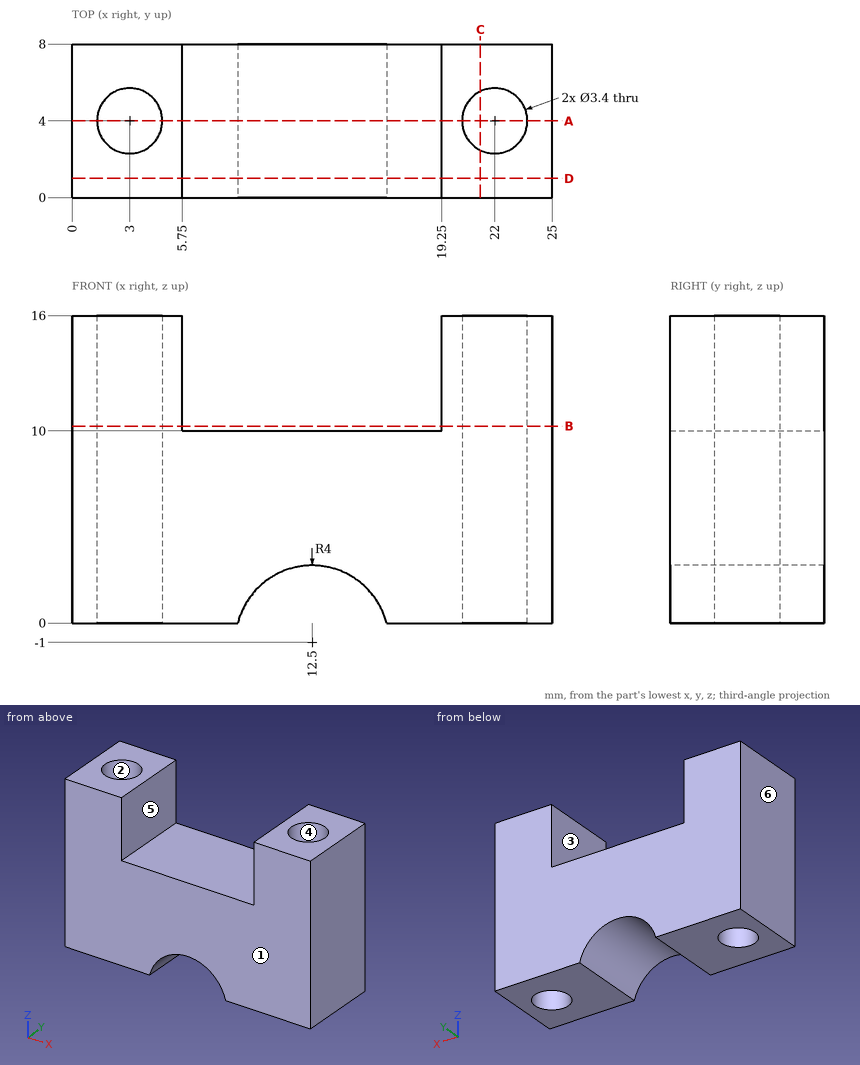
Verification items for this drawing (mm, ordinates from the low corner). A direction names the side the tool comes from. Coordinates: 2 decimals unless noted, no trailing zeros. Loops run counter-clockwise (first coordinate to the right, second up) from the corner with the lowest first, then second, coordinate; pieces in that order, holes last. Notation, with made-up numbers: (55.25, -12.75) -> (76.25, -12.75) arc R17 cw to (76.25, 2.25) -> close; hole circle Ø4 at (17.25, 47). An arc over 180 degrees is marked (long way). Put each result on its own line as item: value.
1. Section check B-B, the plane z = 10.25. Record the boundary of the cut face in (x, y).
Result set:
outline: (0, 0) -> (5.75, 0) -> (5.75, 8) -> (0, 8) -> close; (19.25, 0) -> (25, 0) -> (25, 8) -> (19.25, 8) -> close; hole circle Ø3.4 at (3, 4); hole circle Ø3.4 at (22, 4)
2. Section check C-C, the plane x = 21.25. Record the boundary of the cut face in (y, z).
Result set:
outline: (0, 0) -> (2.47, 0) -> (2.47, 16) -> (0, 16) -> close; (5.53, 0) -> (8, 0) -> (8, 16) -> (5.53, 16) -> close
3. Thickness scan on line 1 (Y direction, x = 22, z = 6.75); line 2 (X direction, y = 2.75, z = 12); line 3 (X direction, y = 1.75, z = 11.25). Record the ranges inside material, lowest first.
Result set:
line 1: y = 0 to 2.3, 5.7 to 8
line 2: x = 0 to 1.85, 4.15 to 5.75, 19.25 to 20.85, 23.15 to 25
line 3: x = 0 to 5.75, 19.25 to 25
4. Mould release check, pull along Y, two halves, no side actions. Record for the marked faces 1, 2, 3 and 4: pulls with the +Y half, pulls with the -Y half, needs draft (parallel to the pull), parting line crosses it, or undercut.
Result set:
face 1: pulls with the -Y half
face 2: undercut
face 3: needs draft
face 4: undercut
5. Section check A-A, the plane y = 4. Record the boundary of the cut face in (x, z).
Result set:
outline: (0, 0) -> (1.3, 0) -> (1.3, 16) -> (0, 16) -> close; (4.7, 0) -> (8.63, 0) arc R4 cw to (16.37, 0) -> (20.3, 0) -> (20.3, 16) -> (19.25, 16) -> (19.25, 10) -> (5.75, 10) -> (5.75, 16) -> (4.7, 16) -> close; (23.7, 0) -> (25, 0) -> (25, 16) -> (23.7, 16) -> close
6. Tool access check on the marked faces 5 and 6. Record the directions out of +Z, -Z, +X, -X, +Y, -Y that give a thin tool (end or side, any length) a straight path to the whole face; none if there is none.
Result set:
face 5: +Z, +Y, -Y
face 6: +Z, -Z, -X, +Y, -Y
7. Section check D-D, the plane y = 1. Record the boundary of the cut face in (x, z).
Result set:
outline: (0, 0) -> (8.63, 0) arc R4 cw to (16.37, 0) -> (25, 0) -> (25, 16) -> (19.25, 16) -> (19.25, 10) -> (5.75, 10) -> (5.75, 16) -> (0, 16) -> close
